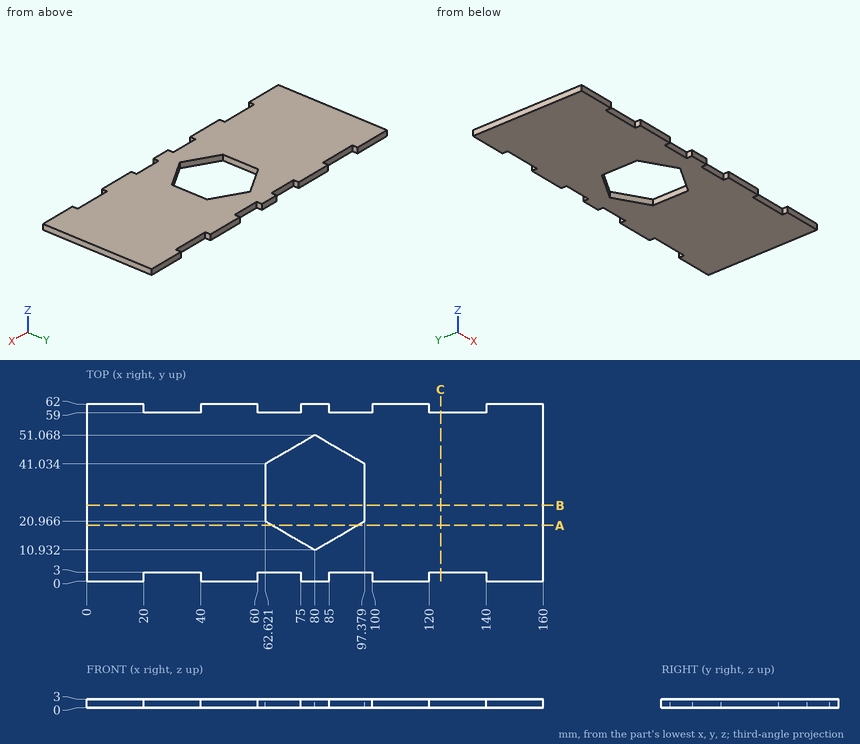
For this review, use the dimensioned drawing (mm, ordinates from the lowest corner) and the shaded views. Give positions to 0.01 mm unless a question says otherwise; leave off trailing zeros. Order: outer loops, then holes, each group sorted by start corner. A loop starts at its lowest first (then second) coordinate and runs counter-clockwise, first axis right, second up. Notation, with made-up numbers: M 25.5,-37.75 L 71.5,-37.75 A18 cw 71.5,-13.75 Z; hole C -24,-18.75 d4. An arc over 180 degrees is marked long. Use one line per item in the form item = value. Start each with the question number.
Item 1: We need section A-A on y = 19.5. Give the boundary of the cut face in (x, z), plus the area to 3 significant figures.
Item 2: Insertion check: pin 1 Ø1.5 at (x, z) = (92.5, 2) entering from +Y; pin 2 Ø10 at (x, y) = (90, 30) entering from +Z. Each pin has a flat end and moves straight along its axis. Give the tip position at first contact, or say it passes through.
Item 3: We need section B-B on y = 26.5. Give the boundary of the cut face in (x, z).
Item 4: To check wall thickness, follow line 1 along X through (y, z) = (27, 1); line 2 along Y through (x, z) = (73, 0.4); line 3 along Y through (x, z) = (95.5, 1.75). State the ranges of each line that lie inside material, in increasing order. Write a range as from..to.
Item 5: We need section C-C on x = 124. Give the boundary of the cut face in (y, z), plus the area to 3 significant figures.
Completed:
q1.outline = M 0,0 L 65.16,0 L 65.16,3 L 0,3 Z; M 94.84,0 L 160,0 L 160,3 L 94.84,3 Z
q1.area = 391 mm²
q2.pin_1 = 59
q2.pin_2 = through
q3.outline = M 0,0 L 62.62,0 L 62.62,3 L 0,3 Z; M 97.38,0 L 160,0 L 160,3 L 97.38,3 Z
q4.line_1 = 0..62.62, 97.38..160
q4.line_2 = 3..14.97, 47.03..59
q4.line_3 = 3..19.88, 42.12..59
q5.outline = M 3,0 L 59,0 L 59,3 L 3,3 Z
q5.area = 168 mm²
